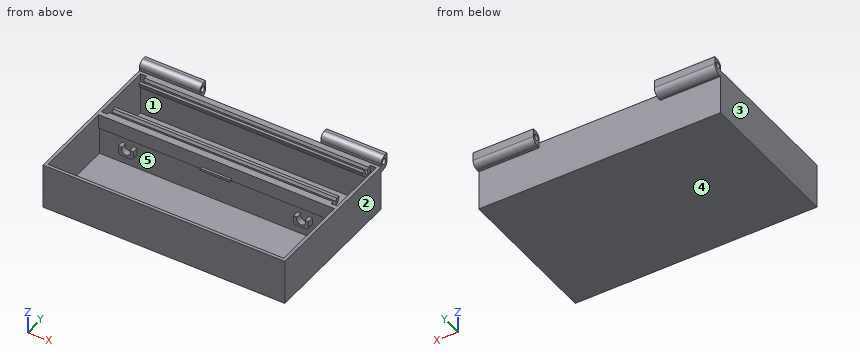
```python
from build123d import *

# Parameters (mm, degrees)
F0_W      = 203.2
F0_H      = 127
F1_DEPTH  = 19.05
F2_T      = -2.54
F3_W      = 198.12
F3_H      = 2.54
F4_DEPTH  = 35.56
F6_DEPTH  = 5.08
F8_DEPTH  = 5.08
F9_R      = 2.54
F10_DEPTH = 50.8
F11_R     = 2.54
F12_DEPTH = 50.8
F14_DEPTH = 198.12
F15_W     = 5
F15_H     = 51.0505303715
F16_DEPTH = 10
F15_H_2   = 2.5
F15_H_3   = 5
F17_DEPTH = 25
F18_W     = 5
F18_H     = 2.5
F18_H_2   = 5
F19_DEPTH = 15
F21_DEPTH = 198.12
F22_W     = 86.5
F22_H     = 3.7755742139
F22_H_2   = 3.4886886767
F23_DEPTH = 15


with BuildPart() as f1:
    # F0 (on Top) → F1 (new body, symmetric)
    with BuildSketch(Plane.XY):
        with Locations((6.5631009638, -9.4094696285)):
            Rectangle(F0_W, F0_H)
    extrude(amount=F1_DEPTH, both=True)

    # F2
    f2_openings = [f1.faces().sort_by_distance(p)[0] for p in [
        (6.563101, -9.40947, 19.05),
    ]]
    offset(amount=F2_T, openings=f2_openings)

    # F3 (on face) → F4 (join, through all)
    with BuildSketch(Plane.XY.offset(-16.51)):
        with Locations((6.5631009638, -1.27)):
            Rectangle(F3_W, F3_H)
    extrude(amount=F4_DEPTH)

    # F5 (on face) → F6 (join)
    with BuildSketch(Plane.XZ.offset(2.54)):
        with BuildLine():
            ThreePointArc((-63.2868990362, -5.842), (-61.490847812, -5.0980512242), (-60.7468990362, -3.302))
            Line((-60.7468990362, -3.302), (-60.7468990362, 1.778))
            Line((-60.7468990362, 1.778), (-63.7272082492, 1.778))
            ThreePointArc((-63.7272082492, 1.778), (-67.0968990362, -3.81), (-70.4665898232, 1.778))
            Line((-70.4665898232, 1.778), (-73.4468990362, 1.778))
            Line((-73.4468990362, 1.778), (-73.4468990362, -3.302))
            ThreePointArc((-73.4468990362, -3.302), (-72.7029502604, -5.0980512242), (-70.9068990362, -5.842))
            Line((-70.9068990362, -5.842), (-63.2868990362, -5.842))
        make_face()
        with BuildLine():
            ThreePointArc((83.5927917508, 1.778), (80.2231009638, -3.81), (76.8534101768, 1.778))
            Line((76.8534101768, 1.778), (73.8731009638, 1.778))
            Line((73.8731009638, 1.778), (73.8731009638, -3.302))
            ThreePointArc((73.8731009638, -3.302), (74.6170497396, -5.0980512242), (76.4131009638, -5.842))
            Line((76.4131009638, -5.842), (84.0331009638, -5.842))
            ThreePointArc((84.0331009638, -5.842), (85.829152188, -5.0980512242), (86.5731009638, -3.302))
            Line((86.5731009638, -3.302), (86.5731009638, 1.778))
            Line((86.5731009638, 1.778), (83.5927917508, 1.778))
        make_face()
    extrude(amount=F6_DEPTH)

    # F7 (on face) → F8 (join)
    with BuildSketch(Plane(origin=(0, -70.3694696285, 0), x_dir=(-1, 0, 0), z_dir=(0, 1, 0))):
        with BuildLine():
            ThreePointArc((-76.8534101768, 1.778), (-80.2231009638, -3.81), (-83.5927917508, 1.778))
            Line((-83.5927917508, 1.778), (-86.5731009638, 1.778))
            Line((-86.5731009638, 1.778), (-86.5731009638, -3.302))
            ThreePointArc((-86.5731009638, -3.302), (-85.829152188, -5.0980512242), (-84.0331009638, -5.842))
            Line((-84.0331009638, -5.842), (-76.4131009638, -5.842))
            ThreePointArc((-76.4131009638, -5.842), (-74.6170497396, -5.0980512242), (-73.8731009638, -3.302))
            Line((-73.8731009638, -3.302), (-73.8731009638, 1.778))
            Line((-73.8731009638, 1.778), (-76.8534101768, 1.778))
        make_face()
        with BuildLine():
            ThreePointArc((60.7468990362, -3.302), (61.490847812, -5.0980512242), (63.2868990362, -5.842))
            Line((63.2868990362, -5.842), (70.9068990362, -5.842))
            ThreePointArc((70.9068990362, -5.842), (72.7029502604, -5.0980512242), (73.4468990362, -3.302))
            Line((73.4468990362, -3.302), (73.4468990362, 1.778))
            Line((73.4468990362, 1.778), (70.4665898232, 1.778))
            ThreePointArc((70.4665898232, 1.778), (67.0968990362, -3.81), (63.7272082492, 1.778))
            Line((63.7272082492, 1.778), (60.7468990362, 1.778))
            Line((60.7468990362, 1.778), (60.7468990362, -3.302))
        make_face()
    extrude(amount=F8_DEPTH)

    # F9 (on face) → F10 (join)
    with BuildSketch(Plane.YZ.offset(108.1631009638)):
        with BuildLine():
            Line((54.0905303715, 21.59), (54.0905303715, 14.7195085883))
            Line((54.0905303715, 14.7195085883), (56.6305303715, 14.7195085883))
            ThreePointArc((56.6305303715, 14.7195085883), (60.22263282, 16.2074061399), (61.7105303715, 19.7995085883))
            Line((61.7105303715, 19.7995085883), (61.7105303715, 26.67))
            Line((61.7105303715, 26.67), (59.1705303715, 26.67))
            ThreePointArc((59.1705303715, 26.67), (55.5784279231, 25.1821024484), (54.0905303715, 21.59))
        make_face()
        with Locations((57.9005303715, 21.59)):
            Circle(F9_R, mode=Mode.SUBTRACT)
    extrude(amount=-F10_DEPTH)

    # F11 (on face) → F12 (join)
    with BuildSketch(Plane(origin=(-95.0368990362, 0, 0), x_dir=(0, -1, 0), z_dir=(-1, 0, 0))):
        with BuildLine():
            Line((-55.3605303715, 13.97), (-54.0905303715, 13.97))
            Line((-54.0905303715, 13.97), (-54.0905303715, 19.05))
            Line((-54.0905303715, 19.05), (-54.0905303715, 21.59))
            ThreePointArc((-54.0905303715, 21.59), (-55.5784279231, 25.1821024484), (-59.1705303715, 26.67))
            Line((-59.1705303715, 26.67), (-61.7105303715, 26.67))
            Line((-61.7105303715, 26.67), (-61.7105303715, 20.32))
            ThreePointArc((-61.7105303715, 20.32), (-59.8506584321, 15.8298719395), (-55.3605303715, 13.97))
        make_face()
        with Locations((-57.9005303715, 21.59)):
            Circle(F11_R, mode=Mode.SUBTRACT)
    extrude(amount=-F12_DEPTH)

    # F13 (on face) → F14 (join, through all)
    with BuildSketch(Plane.YZ.offset(-92.4968990362)):
        with BuildLine():
            Line((46.5505303715, 13.05), (51.5505303715, 13.05))
            Line((51.5505303715, 13.05), (51.5505303715, 19.05))
            Line((51.5505303715, 19.05), (49.0505303715, 19.05))
            Line((49.0505303715, 19.05), (47.8193881256, 16.85))
            ThreePointArc((47.8193881256, 16.85), (46.5163953065, 14.5503884512), (45.3193881256, 16.906906512))
            Line((45.3193881256, 16.906906512), (44.0505303715, 19.05))
            Line((44.0505303715, 19.05), (41.5505303715, 19.05))
            Line((41.5505303715, 19.05), (41.5505303715, 18.05))
            ThreePointArc((41.5505303715, 18.05), (43.0149964656, 14.5144660941), (46.5505303715, 13.05))
        make_face()
        with BuildLine():
            Line((0, 19.05), (0, 13.05))
            Line((0, 13.05), (5, 13.05))
            ThreePointArc((5, 13.05), (8.5355339059, 14.5144660941), (10, 18.05))
            Line((10, 18.05), (10, 19.05))
            Line((10, 19.05), (7.5, 19.05))
            Line((7.5, 19.05), (6.231142246, 16.906906512))
            ThreePointArc((6.231142246, 16.906906512), (5.034135065, 14.5503884512), (3.731142246, 16.85))
            Line((3.731142246, 16.85), (2.5, 19.05))
            Line((2.5, 19.05), (0, 19.05))
        make_face()
    extrude(amount=F14_DEPTH)

    # F15 (on face) → F16 (cut)
    with BuildSketch(Plane.XY.offset(19.05)):
        with Locations((-89.9968990362, 26.0252651858)):
            Rectangle(F15_W, F15_H)
    extrude(amount=-F16_DEPTH, mode=Mode.SUBTRACT)

    # F15 (on face) → F17 (cut)
    with BuildSketch(Plane.XY.offset(19.05)):
        with Locations((-89.9968990362, 50.3005303715)):
            Rectangle(F15_W, F15_H_2)
        with Locations((-89.9968990362, 46.5505303715)):
            Rectangle(F15_W, F15_H_3)
        with Locations((-89.9968990362, 42.8005303715)):
            Rectangle(F15_W, F15_H_2)
    extrude(amount=-F17_DEPTH, mode=Mode.SUBTRACT)

    # F18 (on face) → F19 (cut)
    with BuildSketch(Plane.XY.offset(19.05)):
        with Locations((103.1231009638, 50.3005303715)):
            Rectangle(F18_W, F18_H)
        with Locations((103.1231009638, 46.5505303715)):
            Rectangle(F18_W, F18_H_2)
        with Locations((103.1231009638, 42.8005303715)):
            Rectangle(F18_W, F18_H)
        with Locations((103.1231009638, 8.75)):
            Rectangle(F18_W, F18_H)
        with Locations((103.1231009638, 5)):
            Rectangle(F18_W, F18_H_2)
        with Locations((103.1231009638, 1.25)):
            Rectangle(F18_W, F18_H)
    extrude(amount=-F19_DEPTH, mode=Mode.SUBTRACT)

    # F20 (on face) → F21 (join, through all)
    with BuildSketch(Plane.YZ.offset(-92.4968990362)):
        Polygon((-5.54, 7.05), (-2.54, 7.05), (-2.54, 19.05), (-3.54, 19.05), (-3.54, 9.05), (-5.54, 9.05), align=None)
    extrude(amount=F21_DEPTH)

    # F22 (on face) → F23 (cut)
    with BuildSketch(Plane.XY.offset(19.05)):
        with Locations((-49.2468990362, -5.4277871069)):
            Rectangle(F22_W, F22_H)
        with Locations((62.3731009638, -5.2843443383)):
            Rectangle(F22_W, F22_H_2)
    extrude(amount=-F23_DEPTH, mode=Mode.SUBTRACT)


solid = f1.part
```
For this review, take the finished solid that the model builds, in its own axes (mm). Face numbers are marked on the shaded views. A direction names the side the tool comes from. Coordinates: 2 decimals unless noted, no trailing zeros. Order: outer loops, then holes, each group sorted by start corner. A loop starts at its lowest first (then second) coordinate and runs counter-clockwise, first axis right, second up. Notation, with made-up numbers: (4, -30.75) - (41, -30.75) arc R14 ccw to (41, -6.75) - close; hole circle Ø4 at (27, -12.5). An arc over 180 degrees is marked (long way). Answer as a JSON object with one key per item and string values. Group by question number.
1. The part is to be moulded in two halves that separate along Z. For the marked faces 3, 4 and 5, say which applies: pulls with the +Z half, pulls with the -Z half, needs draft (parallel to the pull), parting line crosses it, or undercut.
2. We need section B-B on z = -11.5. State the section outline as (x, y) points, then the cut area to 3 significant figures.
3. For the marked faces 1 and 2, list the 3-axis set-ups (+Z, -Z, +X, -X, +Y, -Y) from which the entire face can be reached by the end or side of a thin tool; tool diameter is ignored.
4. We need section C-C on y = -25. State the section outline as (x, z) points.
5. For probe 1 along Y at (x, z) = (-46.5, -4); probe 2 along Y at (x, z) = (56, 11); probe 3 along Y at (x, z) = (-14, 19), list the stretches that pass through material, from the lowest coordinate up.
6. We need section A-A on x = 29. State the section outline as (y, z) points.
7. Clearance check with flat-ended pins moving along their axes: P1, Ø4, axis at x = 46, y = 11.5, coming from the +Z side; P2, Ø1.1, axis at x = -24.5, z = 18.5, coming from the +Y side; P3, Ø2.5, axis at x = 85, y = -5.5, coming from the +Z side. State where each tip first meets the part, or that it passes through.
Final values:
{
 "1": {"face 3": "needs draft", "face 4": "pulls with the -Z half", "face 5": "undercut"},
 "2": {"outline": "(-95.04, -72.91) - (108.16, -72.91) - (108.16, 54.09) - (-95.04, 54.09) - close; hole (-92.5, -70.37) - (105.62, -70.37) - (105.62, -2.54) - (-92.5, -2.54) - close; hole (-92.5, 0) - (105.62, 0) - (105.62, 51.55) - (-92.5, 51.55) - close", "area": "2,150 mm²"},
 "3": {"face 1": "none", "face 2": "+Z, -Z, +X, +Y, -Y"},
 "4": {"outline": "(-95.04, -19.05) - (108.16, -19.05) - (108.16, 19.05) - (105.62, 19.05) - (105.62, -16.51) - (-92.5, -16.51) - (-92.5, 19.05) - (-95.04, 19.05) - close"},
 "5": {"probe 1": "-72.91 to -70.37, -2.54 to 0, 51.55 to 54.09", "probe 2": "-72.91 to -70.37, -3.54 to 0, 51.55 to 54.09", "probe 3": "-72.91 to -70.37, -3.54 to 2.53, 7.47 to 10, 41.55 to 44.08, 49.02 to 54.09"},
 "6": {"outline": "(-72.91, -19.05) - (54.09, -19.05) - (54.09, 19.05) - (49.05, 19.05) - (47.82, 16.85) arc R1.5 cw (long way) to (45.32, 16.91) - (44.05, 19.05) - (41.55, 19.05) - (41.55, 18.05) arc R5 ccw to (46.55, 13.05) - (51.55, 13.05) - (51.55, -16.51) - (0, -16.51) - (0, 13.05) - (5, 13.05) arc R5 ccw to (10, 18.05) - (10, 19.05) - (7.5, 19.05) - (6.23, 16.91) arc R1.5 cw (long way) to (3.73, 16.85) - (2.5, 19.05) - (-3.54, 19.05) - (-3.54, 7.05) - (-2.54, 7.05) - (-2.54, -16.51) - (-70.37, -16.51) - (-70.37, 19.05) - (-72.91, 19.05) - close"},
 "7": {"P1": "z = 19.05", "P2": "y = 54.09", "P3": "z = 1.78"}
}
